Could you check a few things on this model? Use its own coordinates, in mm. A direction names the side the tool comes from. Round coordinates to 2 decimals unless told otherwise and drop trailing zeros. Write each loop counter-clockwise with the first axis right and the second up, starting at its lowest first coordinate (ties: lowest second). Pieces come first, ordered by that corner, then holes. Notation, with made-up numbers: (41.25, 23.25) -> (51.25, 23.25) arc R15 ccw to (51.25, 48.25) -> close; hole circle Ø10 at (0.25, 32). An arc over 180 degrees is marked (long way). Answer as CSV lines item,"result". Start each with the question number.
Q1. Imagine slicing it at C-C on z = 2.55. Give the number of separate pieces and of enclosed holes in the cut face, and give its area (3 significant figures).
Q2. If we mould it in two halves opening along Y, with no side actions, what happens to faces 3 (the flat face through (5, -80, 0)), 4 (the flat face through (131.13, -69.24, 2.46)), 5 (the flat face through (145.35, 89.54, 2.46))? For each: pulls with the +Y half, pulls with the -Y half, needs draft (parallel to the pull), parting line crosses it, or undercut.
Q3. If I drill on line 1 (X direction, y = 12.5, z = 4.2); line 2 (Y direction, x = 89.5, z = 3.55); line 3 (Y direction, x = 128.5, z = 0.5), over which ranges is the centre line in solid material (lowest first)? Write a range as [from, to].
Q4. Imagine slicing it at B-B on y = 23. Please give me the cut outline in (x, z).
Q5. Imagine slicing it at A-A on x = 80. Please give me the cut outline in (y, z), and give its area (3 significant figures).
Q6. For faces 1 (the flat face through (-113.38, -83.3, 2.46)), 2 (the flat face through (-98.872, -69.524, 2.465)), which set-ups out of +Z, -Z, +X, -X, +Y, -Y let a thin tool reach every point of the face, with its end or its side?
Q7. Will this pin go through, and if not, where does the flat tip stop? pin 1 Ø3 at (x, y) = (150.99, -24.38) entering from +Z.
from build123d import *

# Parameters (mm, degrees)
SKETCH1_W           = 20
SKETCH1_H           = 80
SKETCH1_R           = 2
SKETCH1_W_2         = 27
SKETCH1_H_2         = 20
SKETCH1_W_3         = 30
SKETCH1_H_3         = 70
SKETCH1_W_4         = 57
BOSS_EXTRUDE1_DEPTH = 5


with BuildPart() as part:
    # Sketch1 → Boss-Extrude1 (new body)
    with BuildSketch(Plane.XY):
        Polygon((-113.154404335, -55.241611667), (-109.012268711, -59.383747291), (-109.012268711, -36.883747291), (-129.012268711, -36.883747291), (-129.012268711, -67.668018539), (-127.296539959, -69.383747291), align=None)
        with Locations((-119.012268711, 3.116252709)):
            Rectangle(SKETCH1_W, SKETCH1_H)
        with Locations((-119.012268711, -26.883747291)):
            Circle(SKETCH1_R, mode=Mode.SUBTRACT)
        with Locations((-119.012268711, 33.116252709)):
            Circle(SKETCH1_R, mode=Mode.SUBTRACT)
        Polygon((-113.154404335, -83.525882915), (-99.012268711, -69.383747291), (-109.012268711, -59.383747291), (-113.154404335, -55.241611667), (-127.296539959, -69.383747291), align=None)
        with Locations((-115.629278069, -66.908873557)):
            Circle(SKETCH1_R, mode=Mode.SUBTRACT)
        Polygon((-84.870133088, -83.525882915), (-89.012268711, -79.383747291), (-99.012268711, -69.383747291), (-113.154404335, -83.525882915), (-99.012268711, -97.668018539), align=None)
        with Locations((-96.537394977, -86.000756649)):
            Circle(SKETCH1_R, mode=Mode.SUBTRACT)
        Polygon((-11.012268711, -79.383747291), (-89.012268711, -79.383747291), (-84.870133088, -83.525882915), (-99.012268711, -97.668018539), (-97.296539959, -99.383747291), (-11.012268711, -99.383747291), align=None)
        with Locations((2.487731289, -89.383747291)):
            Rectangle(SKETCH1_W_2, SKETCH1_H_2)
        with Locations((-1.012268711, -89.383747291)):
            Circle(SKETCH1_R, mode=Mode.SUBTRACT)
        with Locations((30.987731289, -89.383747291)):
            Rectangle(SKETCH1_W_3, SKETCH1_H_2)
        with Locations((35.987731289, -89.383747291)):
            Circle(SKETCH1_R, mode=Mode.SUBTRACT)
        Polygon((116.845595665, -83.525882915), (120.987731289, -79.383747291), (45.987731289, -79.383747291), (45.987731289, -99.383747291), (129.272002536, -99.383747291), (130.987731289, -97.668018539), align=None)
        Polygon((130.987731289, -69.383747291), (120.987731289, -79.383747291), (116.845595665, -83.525882915), (130.987731289, -97.668018539), (145.129866912, -83.525882915), align=None)
        with Locations((128.512857554, -86.000756649)):
            Circle(SKETCH1_R, mode=Mode.SUBTRACT)
        Polygon((140.987731289, -59.383747291), (130.987731289, -69.383747291), (145.129866912, -83.525882915), (159.272002536, -69.383747291), (145.129866912, -55.241611667), align=None)
        with Locations((147.604740646, -66.908873557)):
            Circle(SKETCH1_R, mode=Mode.SUBTRACT)
        Polygon((140.987731289, -31.883747291), (140.987731289, -59.383747291), (145.129866912, -55.241611667), (159.272002536, -69.383747291), (160.987731289, -67.668018539), (160.987731289, -31.883747291), align=None)
        with Locations((150.987731289, 3.116252709)):
            Rectangle(SKETCH1_W, SKETCH1_H_3)
        with Locations((150.987731289, -24.383747291)):
            Circle(SKETCH1_R, mode=Mode.SUBTRACT)
        with Locations((150.987731289, 30.616252709)):
            Circle(SKETCH1_R, mode=Mode.SUBTRACT)
        Polygon((145.129866912, 61.474117085), (140.987731289, 65.616252709), (140.987731289, 38.116252709), (160.987731289, 38.116252709), (160.987731289, 73.900523956), (159.272002536, 75.616252709), align=None)
        Polygon((145.129866912, 89.758388333), (130.987731289, 75.616252709), (140.987731289, 65.616252709), (145.129866912, 61.474117085), (159.272002536, 75.616252709), align=None)
        with Locations((147.604740646, 73.141378975)):
            Circle(SKETCH1_R, mode=Mode.SUBTRACT)
        Polygon((116.845595665, 89.758388333), (120.987731289, 85.616252709), (130.987731289, 75.616252709), (145.129866912, 89.758388333), (130.987731289, 103.900523956), align=None)
        with Locations((128.512857554, 92.233262067)):
            Circle(SKETCH1_R, mode=Mode.SUBTRACT)
        Polygon((45.987731289, 105.616252709), (45.987731289, 85.616252709), (120.987731289, 85.616252709), (116.845595665, 89.758388333), (130.987731289, 103.900523956), (129.272002536, 105.616252709), align=None)
        with Locations((17.487731289, 95.616252709)):
            Rectangle(SKETCH1_W_4, SKETCH1_H_2)
        with Locations((-1.012268711, 95.616252709)):
            Circle(SKETCH1_R, mode=Mode.SUBTRACT)
        with Locations((35.987731289, 95.616252709)):
            Circle(SKETCH1_R, mode=Mode.SUBTRACT)
        Polygon((-84.870133088, 89.758388333), (-89.012268711, 85.616252709), (-11.012268711, 85.616252709), (-11.012268711, 105.616252709), (-97.296539959, 105.616252709), (-99.012268711, 103.900523956), align=None)
        Polygon((-99.012268711, 75.616252709), (-89.012268711, 85.616252709), (-84.870133088, 89.758388333), (-99.012268711, 103.900523956), (-113.154404335, 89.758388333), align=None)
        with Locations((-96.537394977, 92.233262067)):
            Circle(SKETCH1_R, mode=Mode.SUBTRACT)
        Polygon((-109.012268711, 65.616252709), (-99.012268711, 75.616252709), (-113.154404335, 89.758388333), (-127.296539959, 75.616252709), (-113.154404335, 61.474117085), align=None)
        with Locations((-115.629278069, 73.141378975)):
            Circle(SKETCH1_R, mode=Mode.SUBTRACT)
        Polygon((-109.012268711, 43.116252709), (-109.012268711, 65.616252709), (-113.154404335, 61.474117085), (-127.296539959, 75.616252709), (-129.012268711, 73.900523956), (-129.012268711, 43.116252709), align=None)
    extrude(amount=BOSS_EXTRUDE1_DEPTH)


solid = part.part
Checks:
1,separate pieces,"1"
1,enclosed holes,"17"
1,area,"16,800 mm^2"
2,face 3,"needs draft"
2,face 4,"undercut"
2,face 5,"pulls with the +Y half"
3,line 1,"[-129.01, -109.01], [140.99, 160.99]"
3,line 2,"[-99.38, -79.38], [85.62, 105.62]"
3,line 3,"[-99.38, -88], [-84, -71.87], [78.1, 90.23], [94.23, 105.62]"
4,outline,"(-129.01, 0) -> (-109.01, 0) -> (-109.01, 5) -> (-129.01, 5) -> close; (140.99, 0) -> (160.99, 0) -> (160.99, 5) -> (140.99, 5) -> close"
5,outline,"(-99.38, 0) -> (-79.38, 0) -> (-79.38, 5) -> (-99.38, 5) -> close; (85.62, 0) -> (105.62, 0) -> (105.62, 5) -> (85.62, 5) -> close"
5,area,"200 mm^2"
6,face 1,"+Z, -Z, -X, -Y"
6,face 2,"+Z, -Z"
7,pin 1,"through"
